from build123d import *

# Parameters (mm, degrees)
CUT_EXTRUDE_1_DEPTH      = 81.199750623
CUT_EXTRUDE_2_DEPTH      = 81.255840909
CUT_EXTRUDE_2_DEPTH_BACK = 81.255840909
SKETCH_3_R               = 1.5
CUT_EXTRUDE_3_DEPTH      = 81.255840909
CUT_EXTRUDE_3_DEPTH_BACK = 81.255840909
SKETCH_4_R               = 1.5


with BuildPart() as part:
    # 草图1 → 旋转7 (revolve)
    with BuildSketch(Plane(origin=(0, 0, 0), x_dir=(0, 0, -1), z_dir=(1, 0, 0))):
        with BuildLine():
            Line((0, 80), (0, -4))
            ThreePointArc((0, -4), (3.645751311, -1.645751311), (3, 2.645751311))
            Line((3, 2.645751311), (3, 73.354248689))
            ThreePointArc((3, 73.354248689), (3.645751311, 77.645751311), (0, 80))
        make_face()
    revolve(axis=Axis((0, -21.628406948, 0), (0, 1, 0)))

    # 草图2 → 切除-拉伸1 (cut, symmetric)
    with BuildSketch(Plane.XY):
        Polygon((2, 85.145201401), (2, 72), (3, 71), (8.111541525, 71), (8.111541525, 85.145201401), align=None)
        Polygon((8.111541525, -9.145201401), (2, -9.145201401), (2, 4), (3, 5), (8.111541525, 5), align=None)
    cut_extrude_1 = extrude(amount=CUT_EXTRUDE_1_DEPTH, both=True, mode=Mode.SUBTRACT)

    # 镜向1: 切除-拉伸1 across plane
    add(cut_extrude_1.mirror(Plane(origin=(0, 0, 0), x_dir=(0, 0, 1), z_dir=(1, 0, 0))), mode=Mode.SUBTRACT)

    # 草图3 → 切除-拉伸2 (cut, two sides: drawn at the far end of the back side and taken through both)
    with BuildSketch(Plane(origin=(2, 0, 0), x_dir=(0, 0, -1), z_dir=(1, 0, 0)).offset(-CUT_EXTRUDE_2_DEPTH_BACK)):
        with Locations(Location((0, 76, 0), (0, 0, 270))):
            Circle(SKETCH_3_R)
    extrude(amount=CUT_EXTRUDE_2_DEPTH + CUT_EXTRUDE_2_DEPTH_BACK, mode=Mode.SUBTRACT)

    # 草图4 → 切除-拉伸3 (cut, two sides: drawn at the far end of the back side and taken through both)
    with BuildSketch(Plane(origin=(2, 0, 0), x_dir=(0, 0, -1), z_dir=(1, 0, 0)).offset(-CUT_EXTRUDE_3_DEPTH_BACK)):
        with Locations(Location((0, 0, 0), (0, 0, 270))):
            Circle(SKETCH_4_R)
    extrude(amount=CUT_EXTRUDE_3_DEPTH + CUT_EXTRUDE_3_DEPTH_BACK, mode=Mode.SUBTRACT)


solid = part.part
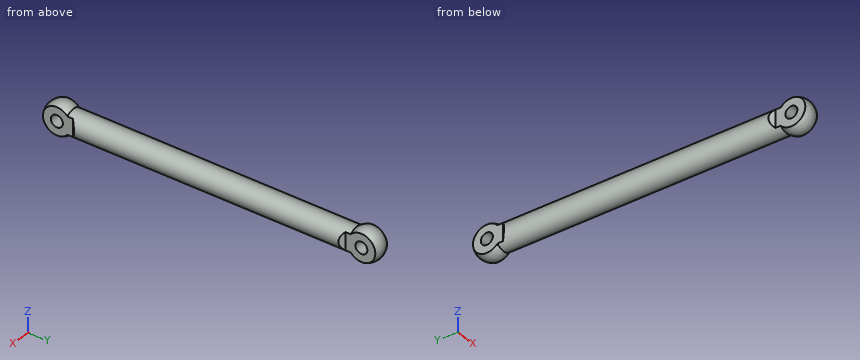
Could you check a few things on this model? Use its own coordinates, in mm. Give positions to 0.01 mm unless a question says otherwise; leave off trailing zeros. Write each loop counter-clockwise with the first axis right and the second up, starting at its lowest first coordinate (ties: lowest second). Pieces come first, ordered by that corner, then holes. Notation, with made-up numbers: (64, 22) -> (107, 22) arc R12 ccw to (107, 28) -> close; hole circle Ø4 at (42, -35.5). An arc over 180 degrees is marked (long way). Answer as a JSON object with one key per item and string values.
Q1. Suppose I cut it at B-B on z = 0. Write out the boundary of the cut face in (x, y).
Taken from the geometry:
{"outline": "(-3, 5) -> (-2, 4) -> (-2, 1.5) -> (2, 1.5) -> (2, 4) -> (3, 5) -> (3, 71) -> (2, 72) -> (2, 74.5) -> (-2, 74.5) -> (-2, 72) -> (-3, 71) -> close; (-2, -3.46) arc R4 ccw to (2, -3.46) -> (2, -1.5) -> (-2, -1.5) -> close; (-2, 77.5) -> (2, 77.5) -> (2, 79.46) arc R4 ccw to (-2, 79.46) -> close"}
Q2. Will these pins go through, and if not, where does the flat tip stop? pin 1 Ø1 at (x, y) = (-1, 42) entering from +Z; pin 2 Ø3.5 at (y, z) = (77, -1) entering from -X; pin 3 Ø3.5 at (y, z) = (-0.5, -1.5) entering from +X.
Taken from the geometry:
{"pin 1": "stops at z = 2.96", "pin 2": "stops at x = -2", "pin 3": "stops at x = 2"}
Q3. Please list where these lines run through material, in increasing order: L1, parallel to Z at x = 0.05, y = 0; L2, parallel to X at y = 19.5, z = -0.25; L3, parallel to X at y = 43, z = -2.
Taken from the geometry:
{"L1": "z = -4 to -1.5, 1.5 to 4", "L2": "x = -2.99 to 2.99", "L3": "x = -2.24 to 2.24"}
Q4. Suppose I cut it at A-A on y = 0. Write out the boundary of the cut face in (x, z), then the cut area to 3 significant figures.
Taken from the geometry:
{"outline": "(-2, -3.46) arc R4 ccw to (2, -3.46) -> (2, -1.5) -> (-2, -1.5) -> close; (-2, 1.5) -> (2, 1.5) -> (2, 3.46) arc R4 ccw to (-2, 3.46) -> close", "area": "18.6 mm²"}
Q5. Suppose I cut it at C-C on x = 0. Write out the boundary of the cut face in (y, z), then the cut area to 3 significant figures.
Taken from the geometry:
{"outline": "(2.65, -3) -> (73.35, -3) arc R4 ccw (long way) to (73.35, 3) -> (2.65, 3) arc R4 ccw (long way) to start; hole circle Ø3 at (0, 0); hole circle Ø3 at (76, 0)", "area": "499 mm²"}
Q6. Suppose I cut it at D-D on y = 11.5. Write out the boundary of the cut face in (x, z).
Taken from the geometry:
{"outline": "circle Ø6 at (0, 0)"}
